Read the model definition and answer for the solid it produces. Units are mm, in the model's axes. Face numbers are marked on the shaded views. A direction names the side the tool comes from. Give positions to 0.01 mm unless a question says otherwise; leave off trailing zeros. Order: outer loops, then holes, each group sorted by start corner. A loop starts at its lowest first (then second) coordinate and runs counter-clockwise, first axis right, second up. Notation, with made-up numbers: M 17,-22 L 50,-22 A29 ccw 50,7 Z; hole C -10.75,47 d11. An arc over 180 degrees is marked long. Write item = value, one per line. Start each with the question number.
from build123d import *
from build123d.topology import SkipClean

# Parameters (mm, degrees)
SKETCH1_R           = 5
BOSS_EXTRUDE1_DEPTH = 20
BOSS_EXTRUDE3_START = 5
BOSS_EXTRUDE3_DEPTH = 5
SKETCH3_R           = 2.5
BOSS_EXTRUDE4_DEPTH = 15
CUT_EXTRUDE2_DEPTH  = 0.1


with BuildPart() as part:
    # Sketch1 → Boss-Extrude1 (new body)
    with BuildSketch(Plane.XY):
        Circle(SKETCH1_R)
    extrude(amount=BOSS_EXTRUDE1_DEPTH)

    # Sketch2 → Boss-Extrude3 (add)
    with SkipClean():  # the faces are left unmerged after this step: merging them gives an invalid solid
        with BuildSketch(Plane(origin=(0, 0, 0), x_dir=(-1, 0, 0), z_dir=(0, 0, -1)).offset(BOSS_EXTRUDE3_START)):
            with BuildLine():
                ThreePointArc((24.874685928, -2.5), (25, 0), (24.874685928, 2.5))
                Line((24.874685928, 2.5), (4.330127019, 2.5))
                ThreePointArc((4.330127019, 2.5), (3.535533906, 3.535533906), (2.5, 4.330127019))
                Line((2.5, 4.330127019), (2.5, 24.874685928))
                ThreePointArc((2.5, 24.874685928), (0, 25), (-2.5, 24.874685928))
                Line((-2.5, 24.874685928), (-2.5, 4.330127019))
                ThreePointArc((-2.5, 4.330127019), (-3.535533906, 3.535533906), (-4.330127019, 2.5))
                Line((-4.330127019, 2.5), (-24.874685928, 2.5))
                ThreePointArc((-24.874685928, 2.5), (-25, 0), (-24.874685928, -2.5))
                Line((-24.874685928, -2.5), (-4.330127019, -2.5))
                ThreePointArc((-4.330127019, -2.5), (-3.535533906, -3.535533906), (-2.5, -4.330127019))
                Line((-2.5, -4.330127019), (-2.5, -24.874685928))
                ThreePointArc((-2.5, -24.874685928), (0, -25), (2.5, -24.874685928))
                Line((2.5, -24.874685928), (2.5, -4.330127019))
                ThreePointArc((2.5, -4.330127019), (3.535533906, -3.535533906), (4.330127019, -2.5))
                Line((4.330127019, -2.5), (24.874685928, -2.5))
            make_face()
        extrude(amount=-BOSS_EXTRUDE3_DEPTH)

    # Sketch3 → Boss-Extrude4 (add)
    with SkipClean():  # the faces are left unmerged after this step: merging them gives an invalid solid
        with BuildSketch(Plane(origin=(0, 0, -5), x_dir=(-1, 0, 0), z_dir=(0, 0, -1))):
            with Locations(Location((-20, 0, 0), (0, 0, 270))):
                Circle(SKETCH3_R)
            with Locations((0, 20)):
                Circle(SKETCH3_R)
            with Locations(Location((20, 0, 0), (0, 0, 270))):
                Circle(SKETCH3_R)
            with Locations((0, -20)):
                Circle(SKETCH3_R)
        extrude(amount=BOSS_EXTRUDE4_DEPTH)

    # Sketch4 → Cut-Extrude2 (cut)
    with SkipClean():  # the faces are left unmerged after this step: merging them gives an invalid solid
        with BuildSketch(Plane.XY.offset(20)):
            Polygon((0.621320344, 2.121320344), (1.159188309, 1.583452378), (1.697056275, 2.121320344), align=None)
            Polygon((1.159188309, 1.583452378), (1.583452378, 1.159188309), (2.121320344, 1.697056275), (2.121320344, 2.121320344), (1.697056275, 2.121320344), align=None)
            Polygon((2.121320344, 1.697056275), (1.583452378, 1.159188309), (2.121320344, 0.621320344), align=None)
            Polygon((0.212132034, 0.212132034), (0, 0), (0.212132034, -0.212132034), (1.583452378, 1.159188309), (1.159188309, 1.583452378), (0, 0.424264069), align=None)
            Polygon((-0.212132034, 0.212132034), (0, 0), (0.212132034, 0.212132034), (0, 0.424264069), align=None)
        extrude(amount=-CUT_EXTRUDE2_DEPTH, mode=Mode.SUBTRACT)


solid = part.part
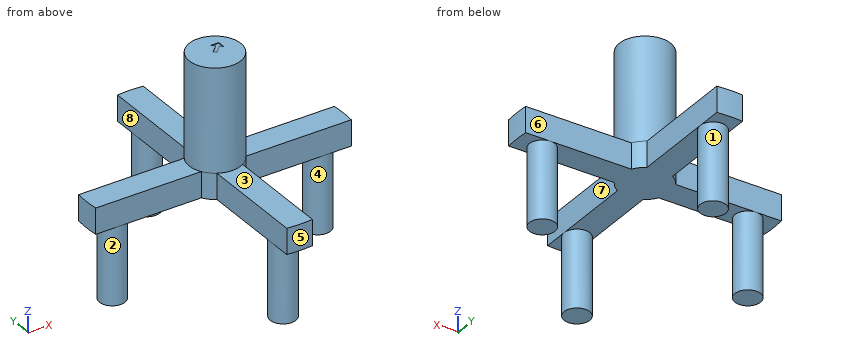
1) Each of these flat-tipped pins is pushed along its axis until it touches: P1, Ø4, axis at x = 13.5, z = -1.5, coming from the +Y side; P2, Ø1.5, axis at y = -17, z = -3.5, coming from the -X side; P3, Ø1.5, axis at x = 15, y = 1, coming from the +Z side. Where does it stop, or does it pass through?
2) Find section D-D on y = 3.5. Determine the outline of the cut face in (x, z), plus the area to 3 significant figures.
3) Find section B-B on y = -15.5. Determine the outline of the cut face in (x, z).
4) Find the intervals of material crossed by probe 1 along X at (y, z) = (0, -16); probe 2 along X at (y, z) = (-14, -2), in increasing order. Write a range as [from, to].
5) Find section A-A on z = -10. Determine the outline of the cut face in (x, y), plus the area to 3 significant figures.
6) For a pull along X with two mould halves and no side action, classify the marked faces 1, 2, 3 and 4 as pulls with the +X half, pulls with the -X half, needs draft (parallel to the pull), parting line crosses it, or undercut.
7) For the marked faces 5, 6, 7 and 8, determine the directions among +Z, -Z, +X, -X, +Y, -Y from which every point of the face is accessible in a straight line to the end or side of a thin tool.
Numbers:
q1.P1 = 2.5
q1.P2 = -2.5
q1.P3 = 0
q2.outline = M -3.57,-5 L 3.57,-5 L 3.57,20 L -3.57,20 Z
q2.area = 179 mm2
q3.outline = M -2.5,-5 L 2.5,-5 L 2.5,0 L -2.5,0 Z
q4.probe_1 = [-22.5, -17.5], [17.5, 22.5]
q4.probe_2 = [-2.5, 2.5]
q5.outline = C -20,0 d5; C 0,-20 d5; C 0,20 d5; C 20,0 d5
q5.area = 78.5 mm2
q6.face_1 = parting line crosses it
q6.face_2 = undercut
q6.face_3 = needs draft
q6.face_4 = undercut
q7.face_5 = +Z, -Z, -Y
q7.face_6 = +Z, -Z, +X, +Y
q7.face_7 = +Z, -Z, +X, -Y
q7.face_8 = +Z, -Z, -X, +Y
